Verification items for this drawing (mm, ordinates from the low corner). A direction names the side the tool comes from. Give positions to 0.01 mm unless a question says otherwise; leave off trailing zeros. Order: outer loops, then holes, each group sorted by start corner. A loop starts at its lowest first (then second) coordinate and runs counter-clockwise, first axis right, second up. Notation, with made-up numbers: M -26,-30 L -6,-30 A18 ccw -6,-7 Z; hole C 69.5,37 d7. An arc over 180 degrees is marked long. Return JSON: item names as keys, results as strings. Group by question number.
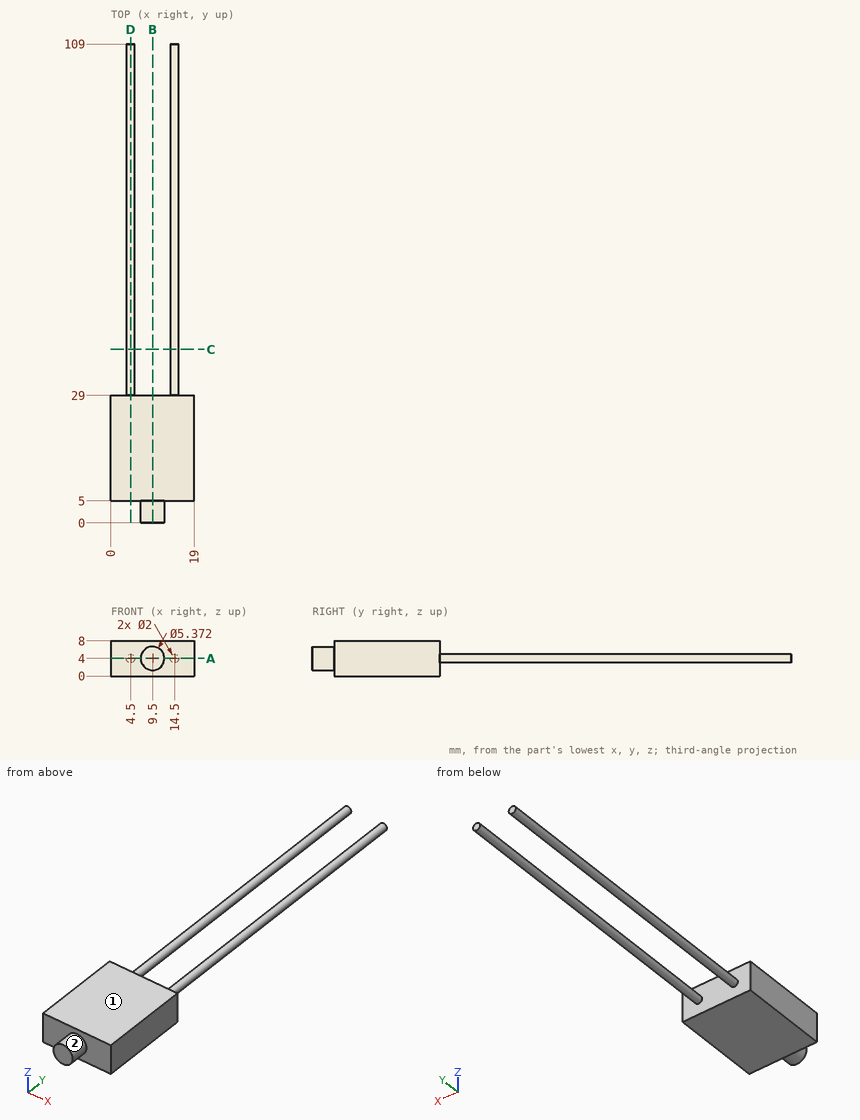
1) Sectioned sample at A-A on z = 4. Record the boundary of the cut face in (x, y), then the cut area to 3 significant figures.
2) Sectioned sample at B-B on x = 9.5. Record the boundary of the cut face in (y, z), then the cut area to 3 significant figures.
3) Sectioned sample at D-D on x = 4.5. Record the boundary of the cut face in (y, z).
4) Depth check by flat-ended pin: P1, Ø8, axis at x = 7, y = 67.5, coming from the +Z side; P2, Ø2, axis at x = 2, y = 42.5, coming from the +Z side; P3, Ø1, axis at x = 5.5, y = 43.5, coming from the -Z side. Enter the tip coordinate at first touch or a pass-through.
5) Material ranges on line 1 along Y through (x, z) = (17.75, 2); line 2 along Y through (x, z) = (7.75, 2.5); line 3 along X through (y, z) = (48, 4.25), recorded low to high.
6) Tool access check on the marked faces 1 and 2. Record the directions out of +Z, -Z, +X, -X, +Y, -Y that give a thin tool (end or side, any length) a straight path to the whole face; none if there is none.
7) Sectioned sample at C-C on y = 39.5. Record the boundary of the cut face in (x, z).
Reply:
{
 "1": {"outline": "M 0,5 L 6.81,5 L 6.81,0 L 12.19,0 L 12.19,5 L 19,5 L 19,29 L 15.5,29 L 15.5,109 L 13.5,109 L 13.5,29 L 5.5,29 L 5.5,109 L 3.5,109 L 3.5,29 L 0,29 Z", "area": "803 mm^2"},
 "2": {"outline": "M 0,1.31 L 5,1.31 L 5,0 L 29,0 L 29,8 L 5,8 L 5,6.69 L 0,6.69 Z", "area": "219 mm^2"},
 "3": {"outline": "M 5,0 L 29,0 L 29,3 L 109,3 L 109,5 L 29,5 L 29,8 L 5,8 Z"},
 "4": {"P1": "z = 5", "P2": "through", "P3": "z = 3.13"},
 "5": {"line 1": "5 to 29", "line 2": "0 to 29", "line 3": "3.53 to 5.47, 13.53 to 15.47"},
 "6": {"face 1": "+Z, +X, -X, +Y, -Y", "face 2": "-Y"},
 "7": {"outline": "C 4.5,4 d2; C 14.5,4 d2"}
}
